Model file for the job. Use its own axes, mm. A direction names the side the tool comes from. Coordinates: 2 decimals unless noted, no trailing zeros. Write each loop counter-clockwise with the first axis right and the second up, starting at its lowest first coordinate (ties: lowest second). Pieces come first, ordered by that corner, then holes.
Q1. Which spindle directions (+Z, -Z, +X, -X, +Y, -Y) get a long thin tool onto all of the face, cutting with end or side? Do faces 1 (the flat face through (12.7, 51, -106)), 2 (the flat face through (135, 10, 0)). Say none if no direction does.
Q2. Pull direction Y, two halves, no side cores. Call faces 3 (the flat face through (279.4, 50, -106)), 4 (the flat face through (144, 0, -113)), 5 (the flat face through (148, 88.9, -106)), 6 (the flat face through (144, 52, -228.6)): released by +Y, released by -Y, zero draft, split by the parting line, or undercut.
Q3. Pin check, flat tips, straight feed: P1, Ø6, axis at x = 199.5, y = 54, coming from the +Z side; P2, Ø4, axis at y = 95.25, z = -88.9, coming from the +X side; P3, Ø4, axis at y = 95.25, z = -139.7, coming from the -X side. Stop position of each tip, or through.
Q4. Band-saw the part on C-C, the plane x = 80. Write the cut outline in (y, z).
Q5. Band-saw the part on A-A, the plane z = -66. Write the cut outline in (x, y).
Q6. Drill centre lines: probe 1 along Y at (x, z) = (27, -114.3); probe 2 along Z at (x, y) = (17, 95.25); probe 3 along X at (y, z) = (45.5, -104). Where is each one in solid material? Low to high.
Q7. Band-saw the part on B-B, the plane y = 50. Write the cut outline in (x, z).
Autodesk Inventor part; units mm, degrees
ref_plane "YZ Plane" through (0, 0, 0) normal (1, 0, 0) x (0, 1, 0)
ref_plane "XZ Plane" through (0, 0, 0) normal (0, 1, 0) x (-1, 0, 0)
ref_plane "XY Plane" through (0, 0, 0) normal (0, 0, 1) x (1, 0, 0)
sketch "BottomBoxFrame" plane through (0, 0, 0) normal (0, 0, 1) x (1, 0, 0)
  line L0 (0, 0) -> (292.1, 0)
  line L1 (292.1, 0) -> (292.1, 101.6)
  line L2 (292.1, 101.6) -> (0, 101.6)
  line L3 (0, 101.6) -> (0, 0)
  dimension "d0" = 101.6
  dimension "d1" = 292.1
extrude "BottomBoxWidth" add sketch "BottomBoxFrame" against normal blind 228.6
sketch "TrayShape" plane through (0, 0, 0) normal (0, 0, 1) x (1, 0, 0)
  line L0 (12.7, 12.7) -> (279.4, 12.7)
  line L1 (279.4, 12.7) -> (279.4, 88.9)
  line L2 (279.4, 88.9) -> (12.7, 88.9)
  line L3 (12.7, 88.9) -> (12.7, 12.7)
  line L4 (0, 0) -> (292.1, 0)
  line L5 (0, 101.6) -> (0, 0)
  line L6 (292.1, 0) -> (292.1, 101.6)
  line L7 (292.1, 101.6) -> (0, 101.6)
  dimension "d5" = 12.7
  dimension "d6" = 12.7
  dimension "d7" = 12.7
  dimension "d10" = 12.7
extrude "TrayCut" cut sketch "TrayShape" against normal blind 215.9 contours L3 L2 L1 L0
sketch "RightHoleGeo" plane through (292.1, 0, 0) normal (1, 0, 0) x (0, 0, -1)
  line L0 (0, 101.6) -> (228.6, 101.6)
  line L1 (0, 0) -> (0, 101.6)
  point P0 (88.9, 95.25)
  point P1 (114.3, 95.25)
  point P2 (139.7, 95.25)
  dimension "d18" = 6.35
  dimension "d19" = 88.9
  dimension "d22" = 25.4
hole "RightPlateHoles" at (292.1, 95.25, -88.9) at (292.1, 95.25, -114.3) at (292.1, 95.25, -139.7) direction (-1, 0, 0) diameter 5.1054 depth 50.8 tip angle 118
sketch "LeftHoleGeo" plane through (0, 0, 0) normal (-1, 0, 0) x (0, 0, 1)
  line L0 (0, 101.6) -> (-228.6, 101.6)
  line L1 (-228.6, 0) -> (-228.6, 101.6)
  point P0 (0, 0)
  point P1 (-139.7, 95.25)
  point P2 (-114.3, 95.25)
  point P3 (-88.9, 95.25)
  dimension "d34" = 6.35
  dimension "d35" = 88.9
  dimension "d38" = 25.4
hole "LeftPlateHoles" at (0, 95.25, -139.7) at (0, 95.25, -114.3) at (0, 95.25, -88.9) direction (1, 0, 0) diameter 5.1054 depth 50.8 tip angle 118
equation "\"d6\" = d5"
equation "\"d7\" = d6"
equation "\"d10\" = d5"
properties part number "BatteryBoxV2-Bottom"
Answer sheet:
1. face 1: +Z
1. face 2: +Z, +X, -X, +Y, -Y
2. face 3: undercut
2. face 4: released by -Y
2. face 5: undercut
2. face 6: zero draft
3. P1: stops at z = -215.9
3. P2: stops at x = 240.97
3. P3: stops at x = 51.13
4. outline: (0, -228.6) - (101.6, -228.6) - (101.6, 0) - (88.9, 0) - (88.9, -215.9) - (12.7, -215.9) - (12.7, 0) - (0, 0) - close
5. outline: (0, 0) - (292.1, 0) - (292.1, 101.6) - (0, 101.6) - close; hole (12.7, 12.7) - (279.4, 12.7) - (279.4, 88.9) - (12.7, 88.9) - close
6. probe 1: y = 0 to 12.7, 88.9 to 92.7, 97.8 to 101.6
6. probe 2: z = -228.6 to -142.25, -137.15 to -116.85, -111.75 to -91.45, -86.35 to 0
6. probe 3: x = 0 to 12.7, 279.4 to 292.1
7. outline: (0, -228.6) - (292.1, -228.6) - (292.1, 0) - (279.4, 0) - (279.4, -215.9) - (12.7, -215.9) - (12.7, 0) - (0, 0) - close
